Verification items for the finished model (mm, model axes). A direction names the side the tool comes from. Coordinates: 2 decimals unless noted, no trailing zeros. Order: outer loops, then holes, each group sorted by start corner. A loop starts at its lowest first (then second) coordinate and runs counter-clockwise, first axis right, second up.
Q1. Draft check along Z on faces 3 (the cylindrical face through (-63.69, 80.05, -6.83)), 4 (the cylindrical face through (164.4, 11.59, 15.12)), 5 (the flat face through (304.8, 12.4, -4)). Enter one of: pulls with the +Z half, pulls with the -Z half, needs draft (parallel to the pull), parting line crosses it, or undercut.
Q2. Thickness scan on line 1 (Y direction, x = 87, z = 0); line 2 (Y direction, x = 271, z = -11.5). Record the ranges inside material, lowest first.
Q3. Cross-section at B-B, the plane x = 180. Record the boundary of the cut face in (y, z).
Q4. Set-up check for faces 1 (the flat face through (-83.706, 157.489, -8.556)), 2 (the cylindrical face through (164.4, 12.4, 2.75)): record each of +Z, -Z, +X, -X, +Y, -Y from which the full face is reachable in a straight line by a thin tool's end or side.
Q5. Depth check by flat-ended pin: P1, Ø6, axis at x = 164.5, z = 12.5, coming from the -Y side; P2, Ø6, axis at x = -66.5, z = 14.5, coming from the -Y side; P3, Ø1.5, axis at y = 39, z = -5.5, coming from the -X side. Enter the tip coordinate at first touch or a pass-through.
Q6. Cross-section at A-A, the plane z = 0. Record the boundary of the cut face in (x, y), and give its area (3 significant figures).
from build123d import *

# Parameters (mm, degrees)
SWEEP1_PROFILE_R        = 19.05
CUT_SWEEP1_PROFILE_R    = 12.7
CUT_EXTRUDE1_DEPTH      = 345.85787932
CUT_EXTRUDE1_DEPTH_BACK = 345.85787932
SKETCH46_R              = 3.937
CHAMFER3_SIZE           = 3.556
CHAMFER3_SIZE2          = 4.237875775


with BuildPart() as part:
    # Sweep1: sweep along a path in Sketch1
    with BuildLine(Plane.XY) as sweep1_path:
        Line((304.8, 0), (27.869834361, 0))
        ThreePointArc((27.869834361, 0), (3.4356049, 6.26228081), (-14.974451087, 23.505179896))
        Line((-14.974451087, 23.505179896), (-95.531870364, 149.954999066))
    # Sweep1 profile (on start of the path) → Sweep1 (sweep)
    with BuildSketch(Plane(origin=(304.8, 0, 0), x_dir=(0, 0, -1), z_dir=(-1, 0, 0))):
        Circle(SWEEP1_PROFILE_R)
    sweep(path=sweep1_path.line)

    # Cut-Sweep1: sweep along a path in Sketch1<2>
    with BuildLine(Plane.XY) as cut_sweep1_path:
        Line((304.8, 0), (27.869834361, 0))
        ThreePointArc((27.869834361, 0), (3.4356049, 6.26228081), (-14.974451087, 23.505179896))
        Line((-14.974451087, 23.505179896), (-95.531870364, 149.954999066))
    # Cut-Sweep1 profile (on start of the path) → Cut-Sweep1 (sweep, cut)
    with BuildSketch(Plane(origin=(304.8, 0, 0), x_dir=(0, 0, -1), z_dir=(-1, 0, 0))):
        Circle(CUT_SWEEP1_PROFILE_R)
    sweep(path=cut_sweep1_path.line, mode=Mode.SUBTRACT)

    # Sketch46 → Cut-Extrude1 (cut, two sides: drawn at the far end of the back side and taken through both)
    with BuildSketch(Plane.XY.offset(-CUT_EXTRUDE1_DEPTH_BACK)):
        with Locations((-23.435845319, 36.786908385)):
            Circle(SKETCH46_R)
    extrude(amount=CUT_EXTRUDE1_DEPTH + CUT_EXTRUDE1_DEPTH_BACK, mode=Mode.SUBTRACT)

    # Chamfer3
    chamfer3_edges = [part.edges().sort_by_distance(p)[0] for p in [
        (-95.531870364, 149.954999066, 12.7),
    ]]
    chamfer3_side = [part.faces().sort_by_distance(p)[0] for p in [
        (-95.531870364, 149.954999066, 18.511184633),
    ]]
    chamfer(chamfer3_edges, length=CHAMFER3_SIZE, length2=CHAMFER3_SIZE2, reference=chamfer3_side[0])


solid = part.part
Check values:
1. face 3: undercut
1. face 4: parting line crosses it
1. face 5: needs draft
2. line 1: y = -19.05 to -12.7, 12.7 to 19.05
2. line 2: y = -15.19 to -5.39, 5.39 to 15.19
3. outline: circle Ø38.1 at (0, 0); hole circle Ø25.4 at (0, 0)
4. face 1: +Z, -Z, -X, +Y
4. face 2: +X
5. P1: stops at y = -16.51
5. P2: stops at y = 74.1
5. P3: stops at x = -47.01
6. outline: (-111.6, 139.72) - (-31.04, 13.27) arc R69.85 ccw to (27.87, -19.05) - (304.8, -19.05) - (304.8, -12.7) - (27.87, -12.7) arc R63.5 cw to (-25.69, 16.68) - (-103.97, 139.56) - (-109.24, 141.22) - close; (-82.54, 153.2) - (-4.26, 30.33) arc R38.1 ccw to (27.87, 12.7) - (304.8, 12.7) - (304.8, 19.05) - (27.87, 19.05) arc R31.75 cw to (1.09, 33.74) - (-79.47, 160.19) - (-81.82, 158.69) - close
6. area: 6,050 mm2
